Source: CAD feature listing. Evaluate the final solid. Frame: model axes, mm. A direction names the side the tool comes from. Coordinates: 2 decimals unless noted, no trailing zeros. Order: outer loops, then holes, each group sorted by start corner. A loop starts at its lowest first (then second) coordinate and runs counter-clockwise, first axis right, second up.
Item 1: Section C-C on x = -21.5. Return the cut outline in (y, z), then the cut area to 3 significant figures.
Item 2: Section D-D on z = 1.6. State how many separate pieces and enclosed holes the cut face has, then the cut area to 3 significant figures.
Item 3: Mould query, pull axis X, two halves, no side actions, for faces 3 (the flat face through (35, 0, 1)), 4 (the flat face through (-35, 0, 1)), 5 (the flat face through (-22.5, 15, 1)). Classes: released by +X, released by -X, zero draft, split by the parting line, or undercut.
Item 4: Section A-A on x = 0. Return the cut outline in (y, z), then the cut area to 3 significant figures.
Item 5: Section B-B on y = 2. Return the cut outline in (x, z), then the cut area to 3 significant figures.
Item 6: Ray query, line 1 (X direction, y = -0.5, z = 0.45); line 2 (Y direction, x = 0, z = 1.5); line 3 (Y direction, x = 26, z = 1.8). Return the intervals inside material, ascending.
Item 7: Contact query for a flat-ended pin moving along its axis: P1, Ø4, axis at x = -7.5, y = -10, coming from the -Z side. Output: stop coordinate, or through.
Item 8: Reachability of faces 1 (the flat face through (22.5, -15, 1)), 2 (the flat face through (0, 5, 0)) from +Z, -Z, +X, -X, +Y, -Y: full face, straight path, thin tool, end or side. Return the list, or none.
from build123d import *

# Parameters (mm, degrees)
SKETCH_W   = 70
SKETCH_H   = 40
SKETCH_R   = 4.2
SKETCH_W_2 = 5
SKETCH_H_2 = 2
SKETCH_W_3 = 4
SKETCH_H_3 = 3
PAD_DEPTH  = 3


with BuildPart() as part:
    # Sketch → Pad (new body)
    with BuildSketch(Plane.XY):
        Rectangle(SKETCH_W, SKETCH_H)
        Circle(SKETCH_R, mode=Mode.SUBTRACT)
        with Locations((-25, 15)):
            Rectangle(SKETCH_W_2, SKETCH_H_2, mode=Mode.SUBTRACT)
        with Locations((25, 15)):
            Rectangle(SKETCH_W_2, SKETCH_H_2, mode=Mode.SUBTRACT)
        with Locations((25, -15)):
            Rectangle(SKETCH_W_2, SKETCH_H_2, mode=Mode.SUBTRACT)
        with Locations((-25, -15)):
            Rectangle(SKETCH_W_2, SKETCH_H_2, mode=Mode.SUBTRACT)
        with Locations((-29, -1.5)):
            Rectangle(SKETCH_W_3, SKETCH_H_3, mode=Mode.SUBTRACT)
        with Locations((-21, -1.5)):
            Rectangle(SKETCH_W_3, SKETCH_H_3, mode=Mode.SUBTRACT)
        with Locations((21, 1.5)):
            Rectangle(SKETCH_W_3, SKETCH_H_3, mode=Mode.SUBTRACT)
        with Locations((29, 1.5)):
            Rectangle(SKETCH_W_3, SKETCH_H_3, mode=Mode.SUBTRACT)
    extrude(amount=PAD_DEPTH)


solid = part.part
Answer list:
1. outline: (-20, 0) - (-3, 0) - (-3, 3) - (-20, 3) - close; (0, 0) - (20, 0) - (20, 3) - (0, 3) - close
1. area: 111 mm2
2. separate pieces: 1
2. enclosed holes: 9
2. area: 2,660 mm2
3. face 3: released by +X
3. face 4: released by -X
3. face 5: undercut
4. outline: (-20, 0) - (-4.2, 0) - (-4.2, 3) - (-20, 3) - close; (4.2, 0) - (20, 0) - (20, 3) - (4.2, 3) - close
4. area: 94.8 mm2
5. outline: (-35, 0) - (-3.69, 0) - (-3.69, 3) - (-35, 3) - close; (3.69, 0) - (19, 0) - (19, 3) - (3.69, 3) - close; (23, 0) - (27, 0) - (27, 3) - (23, 3) - close; (31, 0) - (35, 0) - (35, 3) - (31, 3) - close
5. area: 164 mm2
6. line 1: x = -35 to -31, -27 to -23, -19 to -4.17, 4.17 to 35
6. line 2: y = -20 to -4.2, 4.2 to 20
6. line 3: y = -20 to -16, -14 to 14, 16 to 20
7. P1: stops at z = 0
8. face 1: +Z, -Z
8. face 2: -Z, +X, -X, +Y, -Y
